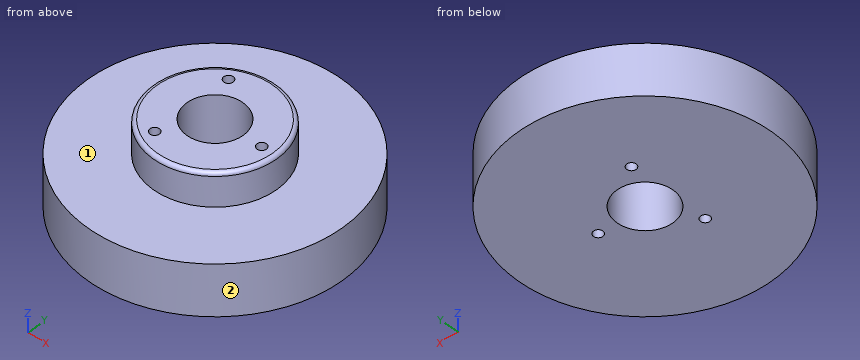
from build123d import *

# Parameters (mm, degrees)
SKETCH_1_R          = 34
EXTRUDE_1_DEPTH     = 13.6
SKETCH_2_R          = 16.5
EXTRUDE_2_DEPTH     = 8.9
FILLET_1_R          = 1
SKETCH_3_R          = 4
CUT_EXTRUDE_1_DEPTH = 54.087192429
SKETCH_4_R          = 7.5
CUT_EXTRUDE_2_DEPTH = 54.087192429
M3X0_52_D           = 2.5


with BuildPart() as part:
    # Эскиз1 → Бобышка-Вытянуть1 (new body)
    with BuildSketch(Plane.XY):
        Circle(SKETCH_1_R)
    extrude(amount=EXTRUDE_1_DEPTH)

    # Эскиз2 → Бобышка-Вытянуть2 (add)
    with BuildSketch(Plane.XY.offset(13.6)):
        Circle(SKETCH_2_R)
    extrude(amount=EXTRUDE_2_DEPTH)

    # Скругление1
    fillet_1_edges = [part.edges().sort_by_distance(p)[0] for p in [
        (-16.5, 0, 22.5),
    ]]
    fillet(fillet_1_edges, radius=FILLET_1_R)

    # Эскиз3 → Вырез-Вытянуть1 (cut, through all)
    with BuildSketch(Plane(origin=(0, 0, 0), x_dir=(-1, 0, 0), z_dir=(0, 0, -1))):
        Circle(SKETCH_3_R)
    extrude(amount=-CUT_EXTRUDE_1_DEPTH, mode=Mode.SUBTRACT)

    # Эскиз4 → Вырез-Вытянуть2 (cut, through all)
    with BuildSketch(Plane.XY.offset(22.5)):
        Circle(SKETCH_4_R)
    extrude(amount=-CUT_EXTRUDE_2_DEPTH, mode=Mode.SUBTRACT)

    # Отверстие обработанное метчиком M3x0.52 (through all)
    with Locations(Plane.XY.offset(22.5)):
        with Locations((-6.25, 10.825317547), (-6.25, -10.825317547), (12.5, 0)):
            Hole(M3X0_52_D / 2)


solid = part.part
Here's how the part is built. I have some questions about the finished solid (model axes, mm). Face numbers are marked on the shaded views. A direction names the side the tool comes from. Coordinates: 2 decimals unless noted, no trailing zeros. Write each loop counter-clockwise with the first axis right and the second up, starting at its lowest first coordinate (ties: lowest second). Pieces come first, ordered by that corner, then holes.
Item 1: I want a section at D-D on z = 19. Write out the boundary of the cut face in (x, y).
Item 2: I want a section at C-C on x = -24.5. Write out the boundary of the cut face in (y, z).
Item 3: I want a section at A-A on x = 0. Write out the boundary of the cut face in (y, z), and give its area (3 significant figures).
Item 4: I want a section at B-B on z = 5. Write out the boundary of the cut face in (x, y), and give its area (3 significant figures).
Item 5: On a 3-axis mill with a long thin cutter (end or side, diameter ignored), from which of +Z, -Z, +X, -X, +Y, -Y can I reach the whole of each face in a straight line? I mean the marked faces 1 and 2. Say none if no direction works.
Item 6: If I drill on line 1 (Y direction, x = -6.25, z = 16.5); line 2 (Z direction, x = 10, y = -31); line 3 (Y direction, x = 11.5, z = 13.75), over which ranges is the centre line in solid material (lowest first)?
Item 7: Will these pins go through, and if not, where does the flat tip stop? pin 1 (2 mm diameter, centred on x = -21, z = 7, fed in from -Y); pin 2 (1.5 mm diameter, centred on y = -15.5, z = 7, fed in from -X); pin 3 (2 mm diameter, centred on x = -6.25, y = -10.83, fed in from +Z); pin 4 (1 mm diameter, centred on y = -19, z = 4, fed in from +X).
Findings below:
1. outline: circle Ø33 at (0, 0); hole circle Ø2.5 at (-6.25, -10.83); hole circle Ø15 at (0, 0); hole circle Ø2.5 at (-6.25, 10.83); hole circle Ø2.5 at (12.5, 0)
2. outline: (-23.57, 0) - (23.57, 0) - (23.57, 13.6) - (-23.57, 13.6) - close
3. outline: (-34, 0) - (-7.5, 0) - (-7.5, 22.5) - (-15.5, 22.5) arc R1 ccw to (-16.5, 21.5) - (-16.5, 13.6) - (-34, 13.6) - close; (7.5, 0) - (34, 0) - (34, 13.6) - (16.5, 13.6) - (16.5, 21.5) arc R1 ccw to (15.5, 22.5) - (7.5, 22.5) - close
3. area: 881 mm2
4. outline: circle Ø68 at (0, 0); hole circle Ø2.5 at (-6.25, -10.83); hole circle Ø15 at (0, 0); hole circle Ø2.5 at (-6.25, 10.83); hole circle Ø2.5 at (12.5, 0)
4. area: 3,440 mm2
5. face 1: +Z
5. face 2: +Z, -Z
6. line 1: y = -15.27 to -12.08, -9.58 to -4.15, 4.15 to 9.58, 12.08 to 15.27
6. line 2: z = 0 to 13.6
6. line 3: y = -11.83 to -0.75, 0.75 to 11.83
7. pin 1: stops at y = -27.5
7. pin 2: stops at x = -30.63
7. pin 3: passes through
7. pin 4: stops at x = 28.53
